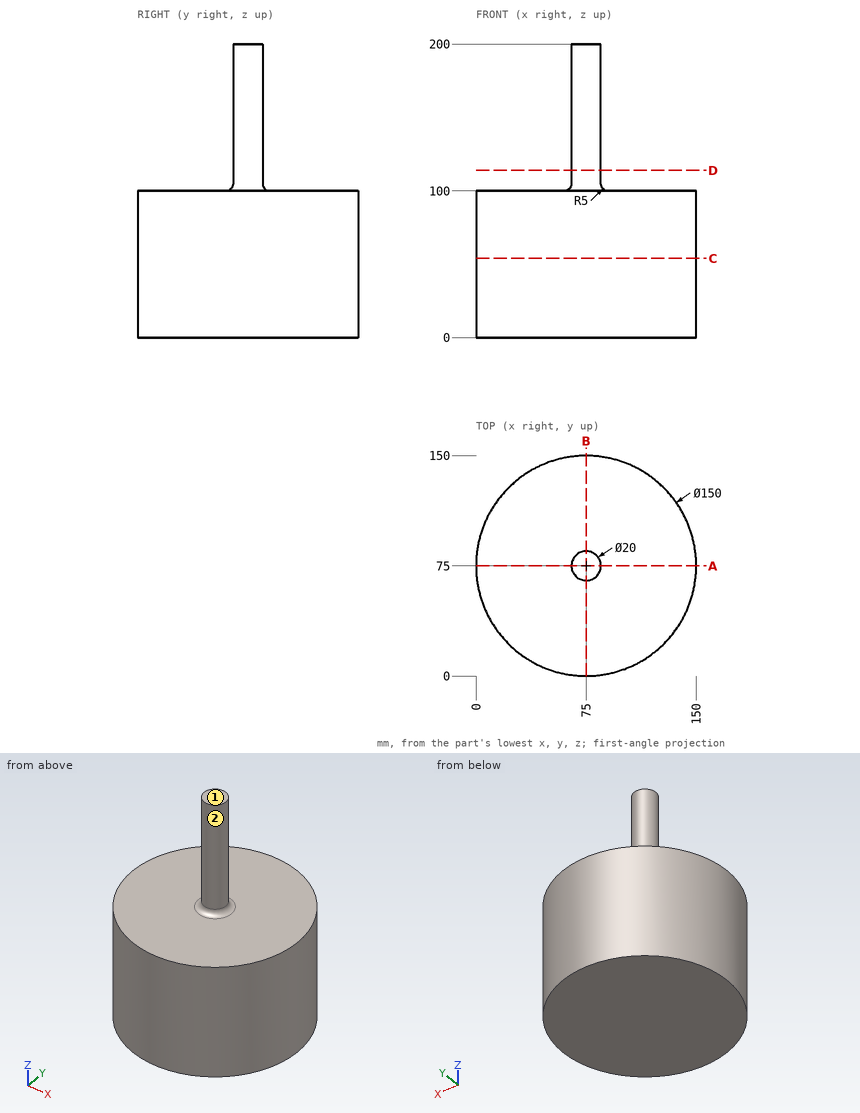
Geometry check sheet. Reference: drawing and pictorial views, mm from the part's lowest x, y, z. A direction names the side the tool comes from. Round coordinates to 2 decimals unless told otherwise and drop trailing zeros. Order: outer loops, then holes, each group sorted by start corner. A loop starts at its lowest first (then second) coordinate and runs counter-clockwise, first axis right, second up. Notation, with made-up numbers: M 65.25,53.25 L 124.25,53.25 A21 ccw 124.25,71.25 Z; hole C -3.5,44.25 d8. An arc over 180 degrees is marked long. Answer as CSV lines item,"result".
1) Sectioned sample at C-C on z = 54. Record the cut outline in (x, y).
Entries:
outline,"C 75,75 d150"
2) Sectioned sample at A-A on y = 75. Record the cut outline in (x, z).
Entries:
outline,"M 0,0 L 150,0 L 150,100 L 90,100 A5 cw 85,105 L 85,200 L 65,200 L 65,105 A5 cw 60,100 L 0,100 Z"
3) Thickness scan on probe 1 along Z at (x, y) = (7, 80); probe 2 along X at (y, z) = (76, 39.5); probe 3 along Y at (x, z) = (72.5, 74). Record the ranges inside material, lowest first. Write a range as [from, to].
Entries:
probe 1,"[0, 100]"
probe 2,"[0.01, 149.99]"
probe 3,"[0.04, 149.96]"
4) Sectioned sample at D-D on z = 114. Record the cut outline in (x, y), and give its area (3 significant figures).
Entries:
outline,"C 75,75 d20"
area,"314 mm2"
5) Tool access check on the marked faces 1 and 2. Record the directions out of +Z, -Z, +X, -X, +Y, -Y that give a thin tool (end or side, any length) a straight path to the whole face; none if there is none.
Entries:
face 1,"+Z, +X, -X, +Y, -Y"
face 2,"+Z"
6) Gauge pin test, flat ends, axial feed: pin 1 Ø5 at (x, z) = (44.5, 62.5) entering from +Y; pin 2 Ø10 at (y, z) = (64, 37.5) entering from +X; pin 3 Ø2 at (x, z) = (128.5, 72) entering from -Y. Record the tip position at first contact, or that the pin passes through.
Entries:
pin 1,"y = 144.58"
pin 2,"x = 149.76"
pin 3,"y = 21.44"
